```python
from build123d import *

# Parameters (mm, degrees)
SKETCH1_W           = 21.59
SKETCH1_H           = 33.02
BOSS_EXTRUDE1_DEPTH = 35.56
BOSS_EXTRUDE2_DEPTH = 8.255


with BuildPart() as part:
    # Sketch1 → Boss-Extrude1 (new body)
    with BuildSketch(Plane(origin=(0, 0, 0), x_dir=(1, 0, 0), z_dir=(0, 1, 0))):
        with Locations((-10.795, 16.51)):
            Rectangle(SKETCH1_W, SKETCH1_H)
    extrude(amount=BOSS_EXTRUDE1_DEPTH)

    # Sketch1_3 → Boss-Extrude2 (add)
    with BuildSketch(Plane(origin=(0, 0, 0), x_dir=(1, 0, 0), z_dir=(0, 1, 0))):
        with BuildLine():
            ThreePointArc((-2.909772, 37.323833597), (-2.057519513, 35.266314085), (0, 34.414061598))
            Line((0, 34.414061598), (0, 33.02))
            Line((0, 33.02), (-21.59, 33.02))
            Line((-21.59, 33.02), (-21.59, 37.323833597))
            Line((-21.59, 37.323833597), (-17.638833597, 41.275))
            Line((-17.638833597, 41.275), (-2.909772, 41.275))
            Line((-2.909772, 41.275), (-2.909772, 37.323833597))
        make_face()
    extrude(amount=BOSS_EXTRUDE2_DEPTH)

    # Mirror1: part across plane


with BuildPart() as part_1:
    add(part.part)
    add(part.part.mirror(Plane(origin=(0, 35.56, 0), x_dir=(1, 0, 0), z_dir=(0, 0, 1))))

    # Mirror2: part across plane


with BuildPart() as part_2:
    add(part_1.part)
    add(part_1.part.mirror(Plane(origin=(0, 35.56, 0), x_dir=(0, 0, 1), z_dir=(-1, 0, 0))))


solid = part_2.part
```
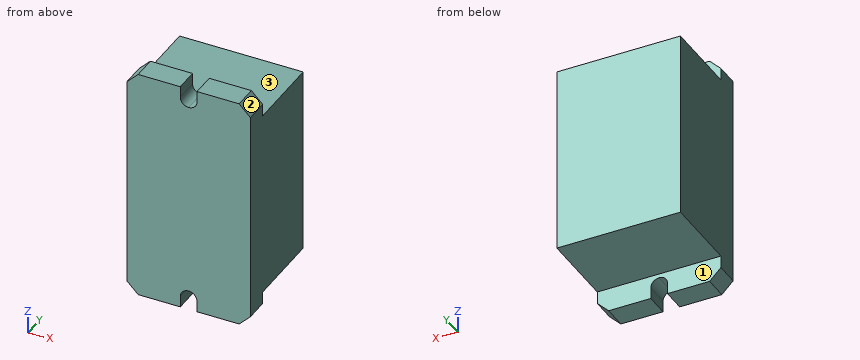
The model under review builds one solid part; all positions refer to its coordinate system, in mm. Face numbers are marked on the shaded views. A direction names the side the tool comes from. Give positions to 0.01 mm unless a question says otherwise; leave off trailing zeros. Order: outer loops, then holes, each group sorted by start corner. A loop starts at its lowest first (then second) coordinate and runs counter-clockwise, first axis right, second up. Notation, with made-up numbers: (82.25, -28) - (135.25, -28) arc R17 cw to (135.25, -14) - close; hole circle Ø6 at (21.5, -20.75). An arc over 180 degrees is marked (long way). Use CSV: the item, a comma, the result in double quotes. Start each with the question number.
Q1. We need section A-A, the plane y = 6.5. Write out the cut boundary in (x, z) (3 decimals), and give its area (3 significant figures).
Q2. We need section B-B, the plane x = 8. Write out the cut boundary in (y, z) (3 decimals), and give its area (3 significant figures).
Q3. Clearance check with flat-ended pins moving along their axes: pin 1 Ø6 at (x, y) = (5.5, 20.5) entering from -Z; pin 2 Ø8 at (x, y) = (1, 22) entering from +Z; pin 3 Ø4 at (x, z) = (9, -36.5) entering from +Y (3 decimals). State where each tip first meets the part, or that it passes through.
Q4. To check wall thickness, follow line 1 along Z through (x, y) = (4, 33.5); line 2 along Y through (x, z) = (-17.5, 37.5) (3 decimals). State the ranges of each line that lie inside material, in increasing order. Write a range as [from, to].
Q5. Tool access review of the marked faces 1, 2 and 3: name each direction out of +Z, -Z, +X, -X, +Y, -Y from which nothing blocks a thin tool from reaching the whole face with its end or side.
Q6. We need section D-D, the plane y = 28. Write out the cut boundary in (x, z).
Q7. We need section C-C, the plane z = 36.5. Write out the cut boundary in (x, y) (3 decimals).
Outcome:
1,outline,"(-21.59, -37.324) - (-17.639, -41.275) - (-2.91, -41.275) - (-2.91, -37.324) arc R2.91 cw to (2.91, -37.324) - (2.91, -41.275) - (17.639, -41.275) - (21.59, -37.324) - (21.59, 37.324) - (17.639, 41.275) - (2.91, 41.275) - (2.91, 37.324) arc R2.91 cw to (-2.91, 37.324) - (-2.91, 41.275) - (-17.639, 41.275) - (-21.59, 37.324) - close"
1,area,"3,460 mm^2"
2,outline,"(0, -41.275) - (8.255, -41.275) - (8.255, -33.02) - (35.56, -33.02) - (35.56, 33.02) - (8.255, 33.02) - (8.255, 41.275) - (0, 41.275) - close"
2,area,"2,480 mm^2"
3,pin 1,"stops at z = -33.02"
3,pin 2,"stops at z = 33.02"
3,pin 3,"stops at y = 8.255"
4,line 1,"z = [-33.02, 33.02]"
4,line 2,"y = [0, 8.255]"
5,face 1,"-Z, +X, -X, +Y"
5,face 2,"+Z, +X, +Y, -Y"
5,face 3,"+Z, +X, -X, +Y"
6,outline,"(-21.59, -33.02) - (21.59, -33.02) - (21.59, 33.02) - (-21.59, 33.02) - close"
7,outline,"(-21.59, 0) - (-2.791, 0) - (-2.791, 8.255) - (-21.59, 8.255) - close; (2.791, 0) - (21.59, 0) - (21.59, 8.255) - (2.791, 8.255) - close"
